Work out the finished part from the listing and answer in its coordinate system (mm). A direction names the side the tool comes from. Coordinates: 2 decimals unless noted, no trailing zeros. Order: outer loops, then holes, each group sorted by start corner. A loop starts at its lowest first (then second) coordinate and runs counter-clockwise, first axis right, second up.
1. A tool of negligible diameter and unlimited length cuts with its end or side. For faces 5 (the flat face through (11.705, 28, -53)), 6 (the flat face through (3, 29.1, -52)), 7 (the flat face through (3, 26.6, 9)), 8 (the flat face through (3, 26.6, -52)), 9 (the flat face through (-6.295, 28, -53)), from which of +Z, -Z, +X, -X, +Y, -Y can it reach the whole face along a straight path? Write none if from no direction.
2. The part is cut by section B-B, the plane z = -28.5. Give the vertices of the cut face in (x, y).
3. The part is cut by section A-A, the plane x = -2.75. Give the vertices of the cut face in (y, z), then the cut area to 3 significant figures.
4. The part is cut by section C-C, the plane y = 9.5. Give the vertices of the cut face in (x, z).
5. Determine the mould class of faces 1 (the flat face through (3, 29.1, 9)), 2 (the cylindrical face through (7.253, 27.833, 7.856)), 3 (the flat face through (-7.295, 18, -22)), 4 (the flat face through (11.705, 28, 10)) for opening direction X: +X half, -X half, draft (parallel to the pull), parting line (faces both ways), or undercut.
6. Find the intervals of material crossed by probe 1 along Y at (x, z) = (5.5, -34); probe 2 along Z at (x, y) = (9, 24.5); probe 3 along Y at (x, z) = (2.75, -52.5), in increasing order.
7. Flat-ended cylindrical pins translate along their axes: pin 1 Ø4 at (x, y) = (-5, 33.5) entering from +Z; pin 2 Ø10 at (x, z) = (-4.5, -26) entering from +Y; pin 3 Ø1.2 at (y, z) = (28, -53.5) entering from +X. Find the tip coordinate at first contact, or state that the pin passes through.
8. The part is cut by section D-D, the plane x = 1.75. Give the vertices of the cut face in (y, z).
Autodesk Inventor part; units mm, degrees
ref_plane "YZ Plane" through (0, 0, 0) normal (1, 0, 0) x (0, 1, 0)
ref_plane "XZ Plane" through (0, 0, 0) normal (0, 1, 0) x (-1, 0, 0)
ref_plane "XY Plane" through (0, 0, 0) normal (0, 0, 1) x (1, 0, 0)
sketch "Sketch5" plane through (0, 0, 0) normal (1, 0, 0) x (0, 1, 0)
  point P0 (0, 0)
sketch "Sketch6" plane through (0, 0, 0) normal (0, 1, 0) x (-1, 0, 0)
  line L0 (7.2949, 6.399) -> (-12.7051, 6.399)
  line L1 (-12.7051, 6.399) -> (-12.7051, -49.101)
  line L2 (-12.7051, -49.101) -> (7.2949, -49.101)
  line L3 (7.2949, -49.101) -> (7.2949, 6.399)
  point P0 (0, 0)
  dimension "d18" = 20
  dimension "d19" = 55.5
extrude "Extrusion4" add sketch "Sketch6" along normal blind 36.1
sketch "Sketch7" plane through (-7.2949, 0, 6.399) normal (0, 0, 1) x (1, 0, 0)
  line L0 (0, 0) -> (0, 36.1)
  line L1 (20, 0) -> (20, 36.1)
  line L2 (1, 26.6) -> (19, 26.6)
  line L3 (19, 26.6) -> (19, 29.1)
  line L4 (19, 29.1) -> (1, 29.1)
  line L5 (1, 29.1) -> (1, 26.6)
  point P0 (7.2949, 0)
  dimension "d25" = 2.5
extrude "Extrusion5" add sketch "Sketch7" along normal blind 7.5
sketch "Sketch8" plane through (12.7051, 0, -49.101) normal (0, 0, -1) x (-1, 0, 0)
  line L0 (0, 0) -> (0, 36.1)
  line L1 (1, 26.6) -> (19, 26.6)
  line L2 (1, 26.6) -> (19, 26.6)
  line L3 (19, 26.6) -> (19, 29.1)
  line L4 (19, 26.6) -> (19, 29.1)
  line L5 (19, 29.1) -> (1, 29.1)
  line L6 (19, 29.1) -> (1, 29.1)
  line L7 (1, 29.1) -> (1, 26.6)
  line L8 (1, 29.1) -> (1, 26.6)
  point P0 (12.7051, 0)
extrude "Extrusion6" add sketch "Sketch8" along normal blind 7.5
sketch "Sketch9" plane through (0, 36.1, 0) normal (0, 1, 0) x (1, 0, 0)
  line L0 (12.7051, -6.399) -> (12.7051, 49.101)
  line L1 (-7.2949, 49.101) -> (-7.2949, -6.399)
  circle A0 centre (2.7051, 40.851) radius 2.95
  line L2 (12.7051, 49.101) -> (-7.2949, 49.101)
  point P0 (0, 0)
  dimension "d35" = 5.9
  dimension "d39" = 10
  dimension "d40" = 8.25
extrude "Extrusion7" add sketch "Sketch9" along normal blind 6
sketch "Sketch11" plane through (-6.2949, 29.1, 6.399) normal (0, 1, 0) x (1, 0, 0)
  line L0 (-1, 0) -> (19, 0)
  line L1 (10, -4) -> (10, 0)
  line L2 (8, -4) -> (8, 0)
  line L3 (10, -4) -> (8, -4)
  line L4 (18, 0) -> (18, -7.5)
  circle A0 centre (13.6676, -4.63) radius 2.25
  circle A1 centre (3.6676, -4.63) radius 2.25
  point P0 (6.2949, 6.399)
  point P1 (0, -7.5)
  dimension "d48" = 4.5
  dimension "d50" = 4.5
hole "Hole1" at (-2.6273, 29.1, 11.029) at (7.3727, 29.1, 11.029) direction (0, -1, 0) diameter 6.35 end through all
sketch "Sketch15" plane through (-6.2949, 29.1, -49.101) normal (0, 1, 0) x (1, 0, 0)
  circle A0 centre (13.6566, 4.6228) radius 2.25
  circle A1 centre (3.6566, 4.6228) radius 2.25
  point P0 (6.2949, -49.101)
  point P1 (18, 0)
  dimension "d64" = 4.5
  dimension "d66" = 4.5
hole "Hole2" at (-2.6383, 29.1, -53.7238) at (7.3617, 29.1, -53.7238) direction (0, -1, 0) diameter 6.35 end through all
properties part number "Serial Motor"
Geometry says:
1. face 5: -Z, +X, +Y, -Y
1. face 6: -Z, +X, -X, +Y
1. face 7: +Z, +X, -X, -Y
1. face 8: -Z, +X, -X, -Y
1. face 9: -Z, -X, +Y, -Y
2. outline: (-7.29, 0) - (12.71, 0) - (12.71, 36.1) - (-7.29, 36.1) - close
3. outline: (0, -49.1) - (26.6, -49.1) - (26.6, -50.55) - (29.1, -50.55) - (29.1, -49.1) - (36.1, -49.1) - (36.1, 6.4) - (29.1, 6.4) - (29.1, 7.86) - (26.6, 7.86) - (26.6, 6.4) - (0, 6.4) - close
3. area: 2,010 mm2
4. outline: (-7.29, -49.1) - (12.71, -49.1) - (12.71, 6.4) - (-7.29, 6.4) - close
5. face 1: draft
5. face 2: undercut
5. face 3: -X half
5. face 4: +X half
6. probe 1: y = 0 to 36.1
6. probe 2: z = -49.1 to 6.4
6. probe 3: y = 26.6 to 29.1
7. pin 1: stops at z = 6.4
7. pin 2: stops at y = 36.1
7. pin 3: stops at x = 11.71
8. outline: (0, -49.1) - (26.6, -49.1) - (26.6, -56.6) - (29.1, -56.6) - (29.1, -49.1) - (36.1, -49.1) - (36.1, -43.64) - (42.1, -43.64) - (42.1, -38.06) - (36.1, -38.06) - (36.1, 6.4) - (29.1, 6.4) - (29.1, 13.9) - (26.6, 13.9) - (26.6, 6.4) - (0, 6.4) - close
